Autodesk Inventor part; units mm, degrees
ref_plane "YZ Plane" through (0, 0, 0) normal (1, 0, 0) x (0, 1, 0)
ref_plane "XY Plane" through (0, 0, 0) normal (0, 0, 1) x (1, 0, 0)
sketch "Skizze1" plane through (0, 0, 0) normal (0, 0, 1) x (1, 0, 0)
  line L0 (-25, -19) -> (25, -19)
  line L1 (25, -19) -> (25, 19)
  line L2 (25, 19) -> (-25, 19)
  line L3 (-25, 19) -> (-25, -19)
  line L4 (-25, -19) -> (25, 19) construction
  line L5 (25, -19) -> (-25, 19) construction
  point P0 (0, 0)
  dimension "d0" = 50
  dimension "d1" = 38
extrude "Extrusion1" add sketch "Skizze1" along normal blind 5
sketch "Skizze2" plane through (0, 0, 5) normal (0, 0, 1) x (1, 0, 0)
  point P0 (0, 0)
ref_plane "Arbeitsebene1" through (0, 19, 0) normal (0, 1, 0) x (-1, 0, 0)
ref_plane "Arbeitsebene2" through (0, -19, 0) normal (0, 1, 0) x (-1, 0, 0)
sketch "Skizze4" plane through (0, 0, 5) normal (0, 0, 1) x (1, 0, 0)
  circle A0 centre (0, 0) radius 10
  circle A1 centre (0, 0) radius 5
  dimension "d12" = 20
  dimension "d13" = 10
extrude "Extrusion2" add sketch "Skizze4" along normal blind 15
ref_plane "Arbeitsebene3" through (0, -10, 0) normal (0, 1, 0) x (-1, 0, 0)
sketch "Skizze5" plane through (0, -10, 0) normal (0, 1, 0) x (-1, 0, 0)
  line L0 (10, 20) -> (-10, 20)
  point P0 (0, 0)
  point P1 (0, 16)
  dimension "d17" = 4
hole "Bohrung1" at (0, -10, 16) direction (0, 1, 0) diameter 3 depth 8 tip angle 118 counterbore diameter 5.68 counterbore depth 2
sketch "Skizze6" plane through (0, -10, 0) normal (0, 1, 0) x (-1, 0, 0)
  point P0 (0, 0)
sketch "Skizze7" plane through (0, 0, 0) normal (0, 0, -1) x (-1, 0, 0)
  circle A0 centre (0, 0) radius 2.5
  dimension "d25" = 5
hole "Bohrung2" at (0, 0, 0) direction (0, 0, 1) diameter 5 depth 5 tip angle 118
properties part number "Laserhalter Unterteil 29112018"
Read the model definition and answer for the solid it produces. Units are mm, in the model's axes. A direction names the side the tool comes from. Coordinates: 2 decimals unless noted, no trailing zeros. Write each loop counter-clockwise with the first axis right and the second up, starting at its lowest first coordinate (ties: lowest second). Pieces come first, ordered by that corner, then holes. Notation, with made-up numbers: (-40, 14) -> (2, 14) arc R11 cw to (2, 20) -> close; hole circle Ø5 at (-26, 26.25). An arc over 180 degrees is marked (long way). Write item = value, one per line.
(1) Section B-B on x = 0 is taken. Write down the section's boundary in (y, z).
From the geometry:
outline = (-19, 0) -> (-2.5, 0) -> (-2.5, 5) -> (-5, 5) -> (-5, 14.5) -> (-8, 14.5) -> (-8, 13.16) -> (-10, 13.16) -> (-10, 5) -> (-19, 5) -> close; (-10, 18.84) -> (-8, 18.84) -> (-8, 17.5) -> (-5, 17.5) -> (-5, 20) -> (-10, 20) -> close; (2.5, 0) -> (19, 0) -> (19, 5) -> (10, 5) -> (10, 20) -> (5, 20) -> (5, 5) -> (2.5, 5) -> close
(2) Straight lines are drawn through the part: L1, parallel to Y at x = 0, z = 10.75; L2, parallel to Z at x = 0, y = -6; L3, parallel to X at y = 0, z = 2.8. For each, find the intervals that lie inside material, in ascending order. Write a range as from..to.
From the geometry:
L1 = -10..-5, 5..10
L2 = 0..14.5, 17.5..20
L3 = -25..-2.5, 2.5..25
(3) Given pin 1 Ø4 at (y, z) = (-2, 8.5) entering from -X; pin 2 Ø4 at (x, z) = (0, 16) entering from +Y; pin 3 Ø6.5 at (x, y) = (0, 0) entering from +Z, each flat-ended and moving along its own axis, determine where each tip first touches the part or whether it passes through.
From the geometry:
pin_1 = -10
pin_2 = 10
pin_3 = 5
(4) Section D-D on z = 10 is taken. Write down the section's boundary in (x, y), plus the area to 3 significant figures.
From the geometry:
outline = circle Ø20 at (0, 0); hole circle Ø10 at (0, 0)
area = 236 mm2
(5) Section C-C on x = -8 is taken. Write down the section's boundary in (y, z).
From the geometry:
outline = (-19, 0) -> (19, 0) -> (19, 5) -> (6, 5) -> (6, 20) -> (-6, 20) -> (-6, 5) -> (-19, 5) -> close
(6) For a pull along Z with two mould halves and no side action, classify faces 4 (the face through (0, 4, 0)), 5 (the face through (1.2, -8, 14.8)), 6 (the face through (-25, 0, 2)) as +Z half, -Z half, draft (parallel to the pull), parting line (faces both ways), or undercut.
From the geometry:
face_4 = -Z half
face_5 = undercut
face_6 = draft
(7) Section A-A on y = 0 is taken. Write down the section's boundary in (x, z), plus the area to 3 significant figures.
From the geometry:
outline = (-25, 0) -> (-2.5, 0) -> (-2.5, 5) -> (-5, 5) -> (-5, 20) -> (-10, 20) -> (-10, 5) -> (-25, 5) -> close; (2.5, 0) -> (25, 0) -> (25, 5) -> (10, 5) -> (10, 20) -> (5, 20) -> (5, 5) -> (2.5, 5) -> close
area = 375 mm2
(8) Which of the six approach directions +Z, -Z, +X, -X, +Y, -Y give full straight-line access (tool end or side, diameter ignored) to faces 1 (the face through (25, 0, 2)), 2 (the face through (-0.85, -8.99, 13.29)), 3 (the face through (-2.17, 9.76, 12.4))?
From the geometry:
face_1 = +Z, -Z, +X, +Y, -Y
face_2 = -Y
face_3 = +Z
